```python
from build123d import *

# Parameters (mm, degrees)
SKETCH2_R             = 1.5
BOSS_EXTRUDE2_DEPTH   = 3
BOSS_EXTRUDE2_2_DEPTH = 3
BOSS_EXTRUDE2_3_DEPTH = 3
BOSS_EXTRUDE2_4_DEPTH = 3
BOSS_EXTRUDE2_5_DEPTH = 3
BOSS_EXTRUDE2_6_DEPTH = 3
BOSS_EXTRUDE2_7_DEPTH = 3
SKETCH3_W             = 48.454319831
SKETCH3_H             = 7.747522056
CUT_EXTRUDE1_DEPTH    = 10


with BuildPart() as part:
    # Sketch2 → Boss-Extrude2 (new body)
    with BuildSketch(Plane(origin=(0, 0, 0), x_dir=(1, 0, 0), z_dir=(0, 1, 0))):
        with Locations(Location((40, 0, 0), (0, 0, 270))):
            Circle(SKETCH2_R)
    extrude(amount=BOSS_EXTRUDE2_DEPTH)


with BuildPart() as body_2:
    # Sketch2 → Boss-Extrude2 2 (new body)
    with BuildSketch(Plane(origin=(0, 0, 0), x_dir=(1, 0, 0), z_dir=(0, 1, 0))):
        with Locations(Location((48, 0, 0), (0, 0, 270))):
            Circle(SKETCH2_R)
    extrude(amount=BOSS_EXTRUDE2_2_DEPTH)


with BuildPart() as body_3:
    # Sketch2 → Boss-Extrude2 3 (new body)
    with BuildSketch(Plane(origin=(0, 0, 0), x_dir=(1, 0, 0), z_dir=(0, 1, 0))):
        with Locations(Location((56, 0, 0), (0, 0, 270))):
            Circle(SKETCH2_R)
    extrude(amount=BOSS_EXTRUDE2_3_DEPTH)


with BuildPart() as body_4:
    # Sketch2 → Boss-Extrude2 4 (new body)
    with BuildSketch(Plane(origin=(0, 0, 0), x_dir=(1, 0, 0), z_dir=(0, 1, 0))):
        with Locations(Location((64, 0, 0), (0, 0, 270))):
            Circle(SKETCH2_R)
    extrude(amount=BOSS_EXTRUDE2_4_DEPTH)


with BuildPart() as body_5:
    # Sketch2 → Boss-Extrude2 5 (new body)
    with BuildSketch(Plane(origin=(0, 0, 0), x_dir=(1, 0, 0), z_dir=(0, 1, 0))):
        with Locations(Location((72, 0, 0), (0, 0, 270))):
            Circle(SKETCH2_R)
    extrude(amount=BOSS_EXTRUDE2_5_DEPTH)


with BuildPart() as body_6:
    # Sketch2 → Boss-Extrude2 6 (new body)
    with BuildSketch(Plane(origin=(0, 0, 0), x_dir=(1, 0, 0), z_dir=(0, 1, 0))):
        with Locations(Location((80, 0, 0), (0, 0, 270))):
            Circle(SKETCH2_R)
    extrude(amount=BOSS_EXTRUDE2_6_DEPTH)


with BuildPart() as body_7:
    # Sketch2 → Boss-Extrude2 7 (new body)
    with BuildSketch(Plane(origin=(0, 0, 0), x_dir=(1, 0, 0), z_dir=(0, 1, 0))):
        with BuildLine():
            Line((0, 4), (32, 4))
            ThreePointArc((32, 4), (36, 0), (32, -4))
            Line((32, -4), (0, -4))
            ThreePointArc((0, -4), (-4, 0), (0, 4))
        make_face()
        with Locations(Location((0, 0, 0), (0, 0, 270))):
            Circle(SKETCH2_R, mode=Mode.SUBTRACT)
        with Locations(Location((8, 0, 0), (0, 0, 270))):
            Circle(SKETCH2_R, mode=Mode.SUBTRACT)
        with Locations(Location((16, 0, 0), (0, 0, 270))):
            Circle(SKETCH2_R, mode=Mode.SUBTRACT)
        with Locations(Location((24, 0, 0), (0, 0, 270))):
            Circle(SKETCH2_R, mode=Mode.SUBTRACT)
        with Locations(Location((32, 0, 0), (0, 0, 270))):
            Circle(SKETCH2_R, mode=Mode.SUBTRACT)
    extrude(amount=BOSS_EXTRUDE2_7_DEPTH)


with BuildPart() as cut_extrude1_tool:
    # Sketch3 → Cut-Extrude1 (new body)
    with BuildSketch(Plane(origin=(0, 0, 0), x_dir=(-1, 0, 0), z_dir=(0, -1, 0))):
        with Locations((-61.501049379, -0.745868802)):
            Rectangle(SKETCH3_W, SKETCH3_H)
    extrude(amount=-CUT_EXTRUDE1_DEPTH)


with BuildPart() as part_1:
    add(part.part)

    # Cut-Extrude1: cut by cut_extrude1_tool
    add(cut_extrude1_tool.part, mode=Mode.SUBTRACT)


with BuildPart() as body_2_1:
    add(body_2.part)

    # Cut-Extrude1: cut by cut_extrude1_tool
    add(cut_extrude1_tool.part, mode=Mode.SUBTRACT)


with BuildPart() as body_3_1:
    add(body_3.part)

    # Cut-Extrude1: cut by cut_extrude1_tool
    add(cut_extrude1_tool.part, mode=Mode.SUBTRACT)


with BuildPart() as body_4_1:
    add(body_4.part)

    # Cut-Extrude1: cut by cut_extrude1_tool
    add(cut_extrude1_tool.part, mode=Mode.SUBTRACT)


with BuildPart() as body_5_1:
    add(body_5.part)

    # Cut-Extrude1: cut by cut_extrude1_tool
    add(cut_extrude1_tool.part, mode=Mode.SUBTRACT)


with BuildPart() as body_6_1:
    add(body_6.part)

    # Cut-Extrude1: cut by cut_extrude1_tool
    add(cut_extrude1_tool.part, mode=Mode.SUBTRACT)


solid = body_7.part
```
Here's how the part is built. I have some questions about the finished solid (model axes, mm). Round coordinates to 2 decimals unless told otherwise and drop trailing zeros. Order: outer loops, then holes, each group sorted by start corner. A loop starts at its lowest first (then second) coordinate and runs counter-clockwise, first axis right, second up. Notation, with made-up numbers: M 23,0.5 L 29,0.5 A10 cw 29,10.5 Z; hole C 76,36 d8. An arc over 180 degrees is marked long. Use CSV: the item, a comma, the result in double quotes.
1) I want a section at B-B (y = 0.4). List the corners of the cut face in (x, z) for me.
Taken from the geometry:
outline,"M 0,-4 L 32,-4 A4 ccw 32,4 L 0,4 A4 ccw Z; hole C 0,0 d3; hole C 8,0 d3; hole C 16,0 d3; hole C 24,0 d3; hole C 32,0 d3"
2) I want a section at D-D (x = 32.5). List the corners of the cut face in (y, z) for me, then the cut area to 3 significant figures.
Taken from the geometry:
outline,"M 0,-3.97 L 3,-3.97 L 3,-1.41 L 0,-1.41 Z; M 0,1.41 L 3,1.41 L 3,3.97 L 0,3.97 Z"
area,"15.3 mm^2"
3) I want a section at A-A (x = 8). List the corners of the cut face in (y, z) for me.
Taken from the geometry:
outline,"M 0,-4 L 3,-4 L 3,-1.5 L 0,-1.5 Z; M 0,1.5 L 3,1.5 L 3,4 L 0,4 Z"
4) If we mould it in two halves opening along Z, with no side actions, what happens to faces 1 (the flat face through (16, 0, -2)), 2 (the cylindrical face through (-4, 1, 0)), 3 (the cylindrical face through (30.536, 1.479, -0.325))? For each: pulls with the +Z half, pulls with the -Z half, needs draft (parallel to the pull), parting line crosses it, or undercut.
Taken from the geometry:
face 1,"needs draft"
face 2,"parting line crosses it"
face 3,"undercut"
5) I'm going to push flat-ended pins straight in: P1, Ø1, axis at y = 1.5, z = -1.5, coming from the +X side; P2, Ø2.5, axis at x = 24, z = 0, coming from the -Y side. Where does each tip first touch, or does it pass through?
Taken from the geometry:
P1,"x = 35.87"
P2,"through"
6) I want a section at C-C (z = -1). List the corners of the cut face in (x, y) for me, then the cut area to 3 significant figures.
Taken from the geometry:
outline,"M -3.87,0 L -1.12,0 L -1.12,3 L -3.87,3 Z; M 1.12,0 L 6.88,0 L 6.88,3 L 1.12,3 Z; M 9.12,0 L 14.88,0 L 14.88,3 L 9.12,3 Z; M 17.12,0 L 22.88,0 L 22.88,3 L 17.12,3 Z; M 25.12,0 L 30.88,0 L 30.88,3 L 25.12,3 Z; M 33.12,0 L 35.87,0 L 35.87,3 L 33.12,3 Z"
area,"85.7 mm^2"
7) I need wall thicknesses on line 1 along X through (y, z) = (2.1, 0); line 2 along X through (y, z) = (2.15, 2.5); line 3 along X through (y, z) = (2.25, 2.75). Which ranges of each line are inside material? Lowest first, please. Write a range as [from, to].
Taken from the geometry:
line 1,"[-4, -1.5], [1.5, 6.5], [9.5, 14.5], [17.5, 22.5], [25.5, 30.5], [33.5, 36]"
line 2,"[-3.12, 35.12]"
line 3,"[-2.9, 34.9]"
